Work out the finished part from the listing and answer in its coordinate system (mm). A direction names the side the tool comes from. Coordinates: 2 decimals unless noted, no trailing zeros. Order: outer loops, then holes, each group sorted by start corner. A loop starts at its lowest first (then second) coordinate and runs counter-clockwise, first axis right, second up. Notation, with made-up numbers: (69.25, -38.5) -> (128.25, -38.5) arc R18 cw to (128.25, -26.5) -> close; hole circle Ø6 at (17.5, 9.5). An arc over 180 degrees is marked (long way). Answer as CSV lines item,"result". Start each with the question number.
Item 1: Each of these flat-tipped pins is pushed along its axis until it touches: pin 1 Ø4.5 at (x, y) = (-49.5, 9) entering from -Z; pin 2 Ø3 at (y, z) = (15, -119.5) entering from -X; pin 3 Ø4 at (x, y) = (-107.5, 1.5) entering from -Z. Where does it stop, or does it pass through?
Item 2: Section A-A (y = 10) is taken. Write down the section's boundary in (x, z).
Item 3: Section C-C (z = -215.5) is taken. Write down the section's boundary in (x, y), then the cut area to 3 significant figures.
Item 4: Which of the six approach directions +Z, -Z, +X, -X, +Y, -Y give full straight-line access (tool end or side, diameter ignored) to faces 4 (the face through (-60, 15, -125)), 5 (the face through (-20, 16, -125)), 6 (the face through (58, 12, -104)), 7 (the face through (60, 7, -109)), 8 (the face through (-95, 15.2, -127.2))?
Item 5: Straight lines are drawn through the part: L1, parallel to Z at x = -27.5, y = 14; L2, parallel to X at y = 12.75, z = -118.5; L3, parallel to Z at x = -50.5, y = 2. For each, find the intervals that lie inside material, in ascending order.
Item 6: For a pull along X with two mould halves and no side action, classify faces 1 (the face through (-115.979, 2.535, -8.555)), 2 (the face through (95, 15.2, -127.2)), 3 (the face through (20, 16, -125)) as pulls with the +X half, pulls with the -X half, needs draft (parallel to the pull), parting line crosses it, or undercut.
Item 7: Section B-B (x = 58) is taken. Write down the section's boundary in (y, z).
```python
from build123d import *

# Parameters (mm, degrees)
BOSS_EXTRUDE1_DEPTH = 125
SKETCH4_W           = 32
SKETCH4_H           = 15
CUT_EXTRUDE1_DEPTH  = 100
SKETCH5_W           = 32
SKETCH5_H           = 15
CUT_EXTRUDE2_DEPTH  = 100
CUT_EXTRUDE3_REACH  = 22
SKETCH6_W           = 30
SKETCH6_H           = 70
CUT_EXTRUDE4_DEPTH  = 15
SKETCH8_R           = 4.5
CUT_EXTRUDE5_DEPTH  = 15
SKETCH9_R           = 5
CUT_EXTRUDE6_DEPTH  = 15
FILLET1_R           = 3
FILLET2_R           = 30
CUT_EXTRUDE7_REACH  = 7
SKETCH11_R          = 1.5
SKETCH11_R_2        = 1.502187573


with BuildPart() as part:
    # Sketch3 → Boss-Extrude1 (new body, symmetric)
    with BuildSketch(Plane(origin=(0, 0, 0), x_dir=(0, 0, -1), z_dir=(1, 0, 0))):
        Polygon((0, 0), (0, 5), (104, 5), (104, 20), (146, 20), (146, 5), (250, 5), (250, 0), align=None)
    extrude(amount=BOSS_EXTRUDE1_DEPTH, both=True)

    # Sketch4 → Cut-Extrude1 (cut)
    with BuildSketch(Plane(origin=(125, 0, 0), x_dir=(0, 0, -1), z_dir=(1, 0, 0))):
        with Locations((125, 7.5)):
            Rectangle(SKETCH4_W, SKETCH4_H)
    extrude(amount=-CUT_EXTRUDE1_DEPTH, mode=Mode.SUBTRACT)

    # Sketch5 → Cut-Extrude2 (cut)
    with BuildSketch(Plane.ZY.offset(125)):
        with Locations((-125, 7.5)):
            Rectangle(SKETCH5_W, SKETCH5_H)
    extrude(amount=-CUT_EXTRUDE2_DEPTH, mode=Mode.SUBTRACT)

    # Sketch6 → Cut-Extrude3 (cut, up to next)
    with BuildSketch(Plane(origin=(0, 20, 0), x_dir=(1, 0, 0), z_dir=(0, 1, 0)), mode=Mode.PRIVATE) as cut_extrude3_sk1:
        with Locations((-110, 125)):
            Rectangle(SKETCH6_W, SKETCH6_H)
    cut_extrude3_tool1 = extrude(cut_extrude3_sk1.sketch, amount=-CUT_EXTRUDE3_REACH, mode=Mode.PRIVATE) & part.part
    add(cut_extrude3_tool1.solids().sort_by_distance((-110, 20, -125))[0], mode=Mode.SUBTRACT)
    # Sketch6 → Cut-Extrude3 (cut, up to next)
    with BuildSketch(Plane(origin=(0, 20, 0), x_dir=(1, 0, 0), z_dir=(0, 1, 0)), mode=Mode.PRIVATE) as cut_extrude3_sk2:
        with Locations((110, 125)):
            Rectangle(SKETCH6_W, SKETCH6_H)
    cut_extrude3_tool2 = extrude(cut_extrude3_sk2.sketch, amount=-CUT_EXTRUDE3_REACH, mode=Mode.PRIVATE) & part.part
    add(cut_extrude3_tool2.solids().sort_by_distance((110, 20, -125))[0], mode=Mode.SUBTRACT)

    # Sketch7 → Cut-Extrude4 (cut)
    with BuildSketch(Plane(origin=(0, 20, 0), x_dir=(1, 0, 0), z_dir=(0, 1, 0))):
        Polygon((0, 146), (-20, 146), (-20, 104), (0, 104), (20, 104), (20, 146), align=None)
    extrude(amount=-CUT_EXTRUDE4_DEPTH, mode=Mode.SUBTRACT)

    # Sketch8 → Cut-Extrude5 (cut)
    with BuildSketch(Plane.ZY.offset(-20)):
        with Locations((-125, 10)):
            Circle(SKETCH8_R)
    extrude(amount=-CUT_EXTRUDE5_DEPTH, mode=Mode.SUBTRACT)

    # Sketch9 → Cut-Extrude6 (cut)
    with BuildSketch(Plane(origin=(-20, 0, 0), x_dir=(0, 0, -1), z_dir=(1, 0, 0))):
        with Locations((125, 10)):
            Circle(SKETCH9_R)
    extrude(amount=-CUT_EXTRUDE6_DEPTH, mode=Mode.SUBTRACT)

    # Fillet1
    fillet1_edges = [part.edges().sort_by_distance(p)[0] for p in [
        (-95, 2.5, -90),
        (-95, 2.5, -160),
        (95, 2.5, -160),
        (95, 2.5, -90),
    ]]
    fillet(fillet1_edges, radius=FILLET1_R)

    # Fillet2
    fillet2_edges = [part.edges().sort_by_distance(p)[0] for p in [
        (-125, 2.5, -250),
        (125, 2.5, 0),
        (-125, 2.5, 0),
        (125, 2.5, -250),
    ]]
    fillet(fillet2_edges, radius=FILLET2_R)

    # Sketch11 → Cut-Extrude7 (cut, up to next)
    with BuildSketch(Plane(origin=(0, 5, 0), x_dir=(1, 0, 0), z_dir=(0, 1, 0)), mode=Mode.PRIVATE) as cut_extrude7_sk1:
        with Locations((-108, 233)):
            Circle(SKETCH11_R)
    cut_extrude7_tool1 = extrude(cut_extrude7_sk1.sketch, amount=-CUT_EXTRUDE7_REACH, mode=Mode.PRIVATE) & part.part
    add(cut_extrude7_tool1.solids().sort_by_distance((-108, 5, -233))[0], mode=Mode.SUBTRACT)
    # Sketch11 → Cut-Extrude7 (cut, up to next)
    with BuildSketch(Plane(origin=(0, 5, 0), x_dir=(1, 0, 0), z_dir=(0, 1, 0)), mode=Mode.PRIVATE) as cut_extrude7_sk2:
        with Locations((108, 233)):
            Circle(SKETCH11_R)
    cut_extrude7_tool2 = extrude(cut_extrude7_sk2.sketch, amount=-CUT_EXTRUDE7_REACH, mode=Mode.PRIVATE) & part.part
    add(cut_extrude7_tool2.solids().sort_by_distance((108, 5, -233))[0], mode=Mode.SUBTRACT)
    # Sketch11 → Cut-Extrude7 (cut, up to next)
    with BuildSketch(Plane(origin=(0, 5, 0), x_dir=(1, 0, 0), z_dir=(0, 1, 0)), mode=Mode.PRIVATE) as cut_extrude7_sk3:
        with Locations((108, 17)):
            Circle(SKETCH11_R)
    cut_extrude7_tool3 = extrude(cut_extrude7_sk3.sketch, amount=-CUT_EXTRUDE7_REACH, mode=Mode.PRIVATE) & part.part
    add(cut_extrude7_tool3.solids().sort_by_distance((108, 5, -17))[0], mode=Mode.SUBTRACT)
    # Sketch11 → Cut-Extrude7 (cut, up to next)
    with BuildSketch(Plane(origin=(0, 5, 0), x_dir=(1, 0, 0), z_dir=(0, 1, 0)), mode=Mode.PRIVATE) as cut_extrude7_sk4:
        with Locations((-108, 17)):
            Circle(SKETCH11_R)
    cut_extrude7_tool4 = extrude(cut_extrude7_sk4.sketch, amount=-CUT_EXTRUDE7_REACH, mode=Mode.PRIVATE) & part.part
    add(cut_extrude7_tool4.solids().sort_by_distance((-108, 5, -17))[0], mode=Mode.SUBTRACT)
    # Sketch11 → Cut-Extrude7 (cut, up to next)
    with BuildSketch(Plane(origin=(0, 5, 0), x_dir=(1, 0, 0), z_dir=(0, 1, 0)), mode=Mode.PRIVATE) as cut_extrude7_sk5:
        with Locations((0, 17)):
            Circle(SKETCH11_R)
    cut_extrude7_tool5 = extrude(cut_extrude7_sk5.sketch, amount=-CUT_EXTRUDE7_REACH, mode=Mode.PRIVATE) & part.part
    add(cut_extrude7_tool5.solids().sort_by_distance((0, 5, -17))[0], mode=Mode.SUBTRACT)
    # Sketch11 → Cut-Extrude7 (cut, up to next)
    with BuildSketch(Plane(origin=(0, 5, 0), x_dir=(1, 0, 0), z_dir=(0, 1, 0)), mode=Mode.PRIVATE) as cut_extrude7_sk6:
        with Locations((0, 233)):
            Circle(SKETCH11_R_2)
    cut_extrude7_tool6 = extrude(cut_extrude7_sk6.sketch, amount=-CUT_EXTRUDE7_REACH, mode=Mode.PRIVATE) & part.part
    add(cut_extrude7_tool6.solids().sort_by_distance((0, 5, -233))[0], mode=Mode.SUBTRACT)


solid = part.part
```
Checked values:
1,pin 1,"stops at z = -146"
1,pin 2,"stops at x = -95"
1,pin 3,"stops at z = -248.1"
2,outline,"(-95, -146) -> (-20, -146) -> (-20, -130) -> (-25, -130) -> (-25, -141) -> (-95, -141) -> close; (-95, -109) -> (-25, -109) -> (-25, -120) -> (-20, -120) -> (-20, -104) -> (-95, -104) -> close; (20, -146) -> (95, -146) -> (95, -141) -> (25, -141) -> (25, -129.5) -> (20, -129.5) -> close; (20, -120.5) -> (25, -120.5) -> (25, -109) -> (95, -109) -> (95, -104) -> (20, -104) -> close"
3,outline,"(-125, 0) -> (125, 0) -> (125, 5) -> (-125, 5) -> close"
3,area,"1,250 mm^2"
4,face 4,"-X, -Y"
4,face 5,"+Z, -Z, +Y"
4,face 6,"+Z, +X, -X, +Y"
4,face 7,"+X, -Y"
4,face 8,"-X, +Y, -Y"
5,L1,"z = -146 to -141, -109 to -104"
5,L2,"x = -25 to -20, 20 to 25"
5,L3,"z = -250 to -141, -109 to 0"
6,face 1,"pulls with the -X half"
6,face 2,"pulls with the +X half"
6,face 3,"undercut"
7,outline,"(0, -250) -> (5, -250) -> (5, -146) -> (20, -146) -> (20, -104) -> (5, -104) -> (5, 0) -> (0, 0) -> (0, -109) -> (15, -109) -> (15, -141) -> (0, -141) -> close"
